```python
from build123d import *

# Parameters (mm, degrees)
SKETCH_1_R      = 1.5
SKETCH_1_R_2    = 1
SKETCH_1_R_3    = 15
SKETCH_1_R_4    = 2.5
SKETCH_1_R_5    = 6.45
EXTRUDE_1_DEPTH = 2
FILLET_1_R      = 0.75


with BuildPart() as part:
    # 草图1 → 凸台-拉伸1 (new body)
    # profile 1 of 11: a face of its own
    with BuildSketch(Plane(origin=(0, 0, 0), x_dir=(1, 0, 0), z_dir=(0, 1, 0))):
        Polygon((-19.848034865, 26.695013128), (-30, 23), (30, 23), (19.848034865, 26.695013128), (0.026493373, 26.695013128), (-0.026493373, 26.695013128), align=None)
    # profile 2 of 11: a face of its own
    with BuildSketch(Plane(origin=(0, 0, 0), x_dir=(1, 0, 0), z_dir=(0, 1, 0))):
        Polygon((-19.848034865, 26.695013128), (-30, 23), (30, 23), (19.848034865, 26.695013128), (0.026493373, 26.695013128), (-0.026493373, 26.695013128), align=None)
    # profile 3 of 11: a face of its own
    with BuildSketch(Plane(origin=(0, 0, 0), x_dir=(1, 0, 0), z_dir=(0, 1, 0))):
        Polygon((-30, 23), (-50, 23), (-50, 7), (-50, -1), (-50, -5), (-50, -23), (-42, -23), (42, -23), (50, -23), (50, -5), (50, -1), (50, 7), (50, 23), (30, 23), align=None)
        with Locations(Location((-46, -15, 0), (0, 0, 270))):
            Circle(SKETCH_1_R, mode=Mode.SUBTRACT)
        with Locations(Location((-30.7465, -13.935, 0), (0, 0, 270))):
            Circle(SKETCH_1_R, mode=Mode.SUBTRACT)
        with Locations(Location((-12.727922061, -5.727922061, 0), (0, 0, 270))):
            Circle(SKETCH_1_R_2, mode=Mode.SUBTRACT)
        with BuildLine():
            ThreePointArc((-20.969611628, -19), (-22.969611628, -17), (-20.969611628, -15))
            Line((-20.969611628, -15), (20.969611628, -15))
            ThreePointArc((20.969611628, -15), (22.969611628, -17), (20.969611628, -19))
            Line((20.969611628, -19), (-20.969611628, -19))
        make_face(mode=Mode.SUBTRACT)
        with Locations(Location((30.7465, -13.935, 0), (0, 0, 270))):
            Circle(SKETCH_1_R, mode=Mode.SUBTRACT)
        with BuildLine():
            ThreePointArc((-6, -13), (-7.5, -11.5), (-6, -10))
            Line((-6, -10), (6, -10))
            ThreePointArc((6, -10), (7.5, -11.5), (6, -13))
            Line((6, -13), (-6, -13))
        make_face(mode=Mode.SUBTRACT)
        with Locations(Location((12.727922061, -5.727922061, 0), (0, 0, 270))):
            Circle(SKETCH_1_R_2, mode=Mode.SUBTRACT)
        with Locations(Location((46, -15, 0), (0, 0, 270))):
            Circle(SKETCH_1_R, mode=Mode.SUBTRACT)
        with Locations(Location((-46, 0, 0), (0, 0, 270))):
            Circle(SKETCH_1_R, mode=Mode.SUBTRACT)
        with Locations(Location((-46, 15, 0), (0, 0, 270))):
            Circle(SKETCH_1_R, mode=Mode.SUBTRACT)
        with Locations(Location((-30.7465, 13.935, 0), (0, 0, 270))):
            Circle(SKETCH_1_R, mode=Mode.SUBTRACT)
        with Locations(Location((-12.727922061, 19.727922061, 0), (0, 0, 270))):
            Circle(SKETCH_1_R_2, mode=Mode.SUBTRACT)
        with Locations((0, 7)):
            Circle(SKETCH_1_R_3, mode=Mode.SUBTRACT)
        with Locations(Location((46, 0, 0), (0, 0, 270))):
            Circle(SKETCH_1_R, mode=Mode.SUBTRACT)
        with Locations(Location((30.7465, 13.935, 0), (0, 0, 270))):
            Circle(SKETCH_1_R, mode=Mode.SUBTRACT)
        with Locations(Location((12.727922061, 19.727922061, 0), (0, 0, 270))):
            Circle(SKETCH_1_R_2, mode=Mode.SUBTRACT)
        with Locations(Location((46, 15, 0), (0, 0, 270))):
            Circle(SKETCH_1_R, mode=Mode.SUBTRACT)
    # profile 4 of 11: a face of its own
    with BuildSketch(Plane(origin=(0, 0, 0), x_dir=(1, 0, 0), z_dir=(0, 1, 0))):
        Polygon((-30, 23), (-50, 23), (-50, 7), (-50, -1), (-50, -5), (-50, -23), (-42, -23), (42, -23), (50, -23), (50, -5), (50, -1), (50, 7), (50, 23), (30, 23), align=None)
        with Locations(Location((-46, -15, 0), (0, 0, 270))):
            Circle(SKETCH_1_R, mode=Mode.SUBTRACT)
        with Locations(Location((-30.7465, -13.935, 0), (0, 0, 270))):
            Circle(SKETCH_1_R, mode=Mode.SUBTRACT)
        with Locations(Location((-12.727922061, -5.727922061, 0), (0, 0, 270))):
            Circle(SKETCH_1_R_2, mode=Mode.SUBTRACT)
        with BuildLine():
            ThreePointArc((-20.969611628, -19), (-22.969611628, -17), (-20.969611628, -15))
            Line((-20.969611628, -15), (20.969611628, -15))
            ThreePointArc((20.969611628, -15), (22.969611628, -17), (20.969611628, -19))
            Line((20.969611628, -19), (-20.969611628, -19))
        make_face(mode=Mode.SUBTRACT)
        with Locations(Location((30.7465, -13.935, 0), (0, 0, 270))):
            Circle(SKETCH_1_R, mode=Mode.SUBTRACT)
        with BuildLine():
            ThreePointArc((-6, -13), (-7.5, -11.5), (-6, -10))
            Line((-6, -10), (6, -10))
            ThreePointArc((6, -10), (7.5, -11.5), (6, -13))
            Line((6, -13), (-6, -13))
        make_face(mode=Mode.SUBTRACT)
        with Locations(Location((12.727922061, -5.727922061, 0), (0, 0, 270))):
            Circle(SKETCH_1_R_2, mode=Mode.SUBTRACT)
        with Locations(Location((46, -15, 0), (0, 0, 270))):
            Circle(SKETCH_1_R, mode=Mode.SUBTRACT)
        with Locations(Location((-46, 0, 0), (0, 0, 270))):
            Circle(SKETCH_1_R, mode=Mode.SUBTRACT)
        with Locations(Location((-46, 15, 0), (0, 0, 270))):
            Circle(SKETCH_1_R, mode=Mode.SUBTRACT)
        with Locations(Location((-30.7465, 13.935, 0), (0, 0, 270))):
            Circle(SKETCH_1_R, mode=Mode.SUBTRACT)
        with Locations(Location((-12.727922061, 19.727922061, 0), (0, 0, 270))):
            Circle(SKETCH_1_R_2, mode=Mode.SUBTRACT)
        with Locations((0, 7)):
            Circle(SKETCH_1_R_3, mode=Mode.SUBTRACT)
        with Locations(Location((46, 0, 0), (0, 0, 270))):
            Circle(SKETCH_1_R, mode=Mode.SUBTRACT)
        with Locations(Location((30.7465, 13.935, 0), (0, 0, 270))):
            Circle(SKETCH_1_R, mode=Mode.SUBTRACT)
        with Locations(Location((12.727922061, 19.727922061, 0), (0, 0, 270))):
            Circle(SKETCH_1_R_2, mode=Mode.SUBTRACT)
        with Locations(Location((46, 15, 0), (0, 0, 270))):
            Circle(SKETCH_1_R, mode=Mode.SUBTRACT)
    # profile 5 of 11: a face of its own
    with BuildSketch(Plane(origin=(0, 0, 0), x_dir=(1, 0, 0), z_dir=(0, 1, 0))):
        with Locations((0, 7)):
            Circle(SKETCH_1_R_3)
        with BuildLine():
            ThreePointArc((13, 7), (12.434860091, 3.208660592), (10.788576229, -0.253042323))
            ThreePointArc((10.788576229, -0.253042323), (9.192388155, -2.192388155), (7.253042323, -3.788576229))
            ThreePointArc((7.253042323, -3.788576229), (0, -6), (-7.253042323, -3.788576229))
            ThreePointArc((-7.253042323, -3.788576229), (-9.192388155, -2.192388155), (-10.788576229, -0.253042323))
            ThreePointArc((-10.788576229, -0.253042323), (-13, 7), (-10.788576229, 14.253042323))
            ThreePointArc((-10.788576229, 14.253042323), (-9.192388155, 16.192388155), (-7.253042323, 17.788576229))
            ThreePointArc((-7.253042323, 17.788576229), (0, 20), (7.253042323, 17.788576229))
            ThreePointArc((7.253042323, 17.788576229), (9.192388155, 16.192388155), (10.788576229, 14.253042323))
            ThreePointArc((10.788576229, 14.253042323), (12.434860091, 10.791339408), (13, 7))
        make_face(mode=Mode.SUBTRACT)
    # profile 6 of 11: a face of its own
    with BuildSketch(Plane(origin=(0, 0, 0), x_dir=(1, 0, 0), z_dir=(0, 1, 0))):
        with BuildLine():
            ThreePointArc((7.253042323, -3.788576229), (9.192388155, -2.192388155), (10.788576229, -0.253042323))
            Line((10.788576229, -0.253042323), (4.242640687, 6.292893219))
            ThreePointArc((4.242640687, 6.292893219), (3.949747468, 7), (4.242640687, 7.707106781))
            Line((4.242640687, 7.707106781), (10.788576229, 14.253042323))
            ThreePointArc((10.788576229, 14.253042323), (9.192388155, 16.192388155), (7.253042323, 17.788576229))
            Line((7.253042323, 17.788576229), (0.707106781, 11.242640687))
            ThreePointArc((0.707106781, 11.242640687), (0, 10.949747468), (-0.707106781, 11.242640687))
            Line((-0.707106781, 11.242640687), (-7.253042323, 17.788576229))
            ThreePointArc((-7.253042323, 17.788576229), (-9.192388155, 16.192388155), (-10.788576229, 14.253042323))
            Line((-10.788576229, 14.253042323), (-4.242640687, 7.707106781))
            ThreePointArc((-4.242640687, 7.707106781), (-3.949747468, 7), (-4.242640687, 6.292893219))
            Line((-4.242640687, 6.292893219), (-10.788576229, -0.253042323))
            ThreePointArc((-10.788576229, -0.253042323), (-9.192388155, -2.192388155), (-7.253042323, -3.788576229))
            Line((-7.253042323, -3.788576229), (-0.707106781, 2.757359313))
            ThreePointArc((-0.707106781, 2.757359313), (0, 3.050252532), (0.707106781, 2.757359313))
            Line((0.707106781, 2.757359313), (7.253042323, -3.788576229))
        make_face()
        with Locations(Location((-3.181980515, 3.818019485, 0), (0, 0, 270))):
            Circle(SKETCH_1_R_2, mode=Mode.SUBTRACT)
        with Locations(Location((-3.181980515, 10.181980515, 0), (0, 0, 270))):
            Circle(SKETCH_1_R_2, mode=Mode.SUBTRACT)
        with Locations(Location((3.181980515, 3.818019485, 0), (0, 0, 270))):
            Circle(SKETCH_1_R_2, mode=Mode.SUBTRACT)
        with Locations(Location((0, 7, 0), (0, 0, 270))):
            Circle(SKETCH_1_R_4, mode=Mode.SUBTRACT)
        with Locations(Location((3.181980515, 10.181980515, 0), (0, 0, 270))):
            Circle(SKETCH_1_R_2, mode=Mode.SUBTRACT)
    # profile 7 of 11: a face of its own
    with BuildSketch(Plane(origin=(0, 0, 0), x_dir=(1, 0, 0), z_dir=(0, 1, 0))):
        Polygon((42, -23), (-42, -23), (-30, -35), (30, -35), align=None)
        with BuildLine():
            ThreePointArc((-20.969611628, -31), (-22.969611628, -29), (-20.969611628, -27))
            Line((-20.969611628, -27), (20.969611628, -27))
            ThreePointArc((20.969611628, -27), (22.969611628, -29), (20.969611628, -31))
            Line((20.969611628, -31), (-20.969611628, -31))
        make_face(mode=Mode.SUBTRACT)
    # profile 8 of 11: a face of its own
    with BuildSketch(Plane(origin=(0, 0, 0), x_dir=(1, 0, 0), z_dir=(0, 1, 0))):
        Polygon((-50, -5), (-50, -1), (-58, 7), (-62, 7), align=None)
    # profile 9 of 11: a face of its own
    with BuildSketch(Plane(origin=(0, 0, 0), x_dir=(1, 0, 0), z_dir=(0, 1, 0))):
        Polygon((-50, 7), (-50, 23), (-66, 23), (-66, 7), (-62, 7), (-58, 7), align=None)
        with Locations(Location((-58, 15, 0), (0, 0, 270))):
            Circle(SKETCH_1_R_5, mode=Mode.SUBTRACT)
    # profile 10 of 11: a face of its own
    with BuildSketch(Plane(origin=(0, 0, 0), x_dir=(1, 0, 0), z_dir=(0, 1, 0))):
        Polygon((66, 23), (50, 23), (50, 7), (58, 7), (62, 7), (66, 7), align=None)
        with Locations(Location((58, 15, 0), (0, 0, 270))):
            Circle(SKETCH_1_R_5, mode=Mode.SUBTRACT)
    # profile 11 of 11: a face of its own
    with BuildSketch(Plane(origin=(0, 0, 0), x_dir=(1, 0, 0), z_dir=(0, 1, 0))):
        Polygon((58, 7), (50, -1), (50, -5), (62, 7), align=None)
    extrude(amount=EXTRUDE_1_DEPTH)

    # 圆角1
    fillet_1_edges = [part.edges().sort_by_distance(p)[0] for p in [
        (66, 1, -23),
        (66, 1, -7),
        (62, 1, -7),
        (50, 1, 5),
        (50, 1, 23),
        (42, 1, 23),
        (30, 1, 35),
        (-30, 1, 35),
        (-42, 1, 23),
        (-50, 1, 23),
        (-50, 1, 5),
        (-62, 1, -7),
        (-66, 1, -7),
        (50, 1, -7),
        (50, 1, 1),
        (58, 1, -7),
        (-50, 1, 1),
        (-50, 1, -7),
        (-58, 1, -7),
    ]]
    fillet(fillet_1_edges, radius=FILLET_1_R)


solid = part.part
```
The model under review builds one solid part; all positions refer to its coordinate system, in mm. A direction names the side the tool comes from. Round coordinates to 2 decimals unless told otherwise and drop trailing zeros. Loops run counter-clockwise (first coordinate to the right, second up) from the corner with the lowest first, then second, coordinate; pieces in that order, holes last. Notation, with made-up numbers: (50, -30) - (66, -30) arc R19 ccw to (66, 6) - close; hole circle Ø4 at (44, 19.25). An arc over 180 degrees is marked (long way). Use a Markdown table: item, result. Add a question column.
Q1. Add section A-A (x = -46). State the section outline as (y, z) points, plus the area to 3 significant figures.
Q2. Add section B-B (y = 1.5). State how many separate pieces and enclosed holes the cut face has, plus the area to 3 significant figures.
Q3. For probe 1 along Z at (x, y) = (11.5, 1.1); probe 2 along Z at (x, y) = (-30, 0.9); probe 3 along X at (y, z) = (0.5, 16), list the stretches that pass through material, from the lowest coordinate up.
Q4. Machinability: for faces 3 (the face through (-4.026, 0.986, 0.561)), 4 (the face through (56, 1, -1)), which of the approach directions +Z, -Z, +X, -X, +Y, -Y give a long, thin tool a straight path to every point of the face, cutting with its end or side? Answer none if there is none.
Q5. The part is to be moulded in two halves that separate along Z. For faces 1 (the face through (-36, 1, 29)), 2 (the face through (44.536, 0.986, -0.325)), say which applies: pulls with the +Z half, pulls with the -Z half, needs draft (parallel to the pull), parting line crosses it, or undercut.
Q6. Insertion check: pin 1 Ø1 at (x, y) = (-49, 1.5) entering from -Z; pin 2 Ø2 at (x, z) = (27.5, 17.5) entering from -Y; pin 3 Ø0.6 at (y, z) = (1, 14.5) entering from -X. Each pin has a flat end and moves straight along its axis. Give the tip position at first contact, or say it passes through.
Worked answers:
| question | item | result |
|---|---|---|
| 1 | outline | (0, -23) - (2, -23) - (2, -16.5) - (0, -16.5) - close; (0, -13.5) - (2, -13.5) - (2, -1.5) - (0, -1.5) - close; (0, 1.5) - (2, 1.5) - (2, 13.5) - (0, 13.5) - close; (0, 16.5) - (2, 16.5) - (2, 23) - (0, 23) - close |
| 1 | area | 74.0 mm² |
| 2 | separate pieces | 1 |
| 2 | enclosed holes | 30 |
| 2 | area | 5,170 mm² |
| 3 | probe 1 | -26.7 to -13.06, -0.94 to 15, 19 to 27, 31 to 35 |
| 3 | probe 2 | -23 to -15.24, -12.63 to 12.63, 15.24 to 34.93 |
| 3 | probe 3 | -50 to -47.12, -44.88 to -22.7, 22.7 to 44.88, 47.12 to 50 |
| 4 | face 3 | +Y, -Y |
| 4 | face 4 | +Z, +X, +Y, -Y |
| 5 | face 1 | pulls with the +Z half |
| 5 | face 2 | undercut |
| 6 | pin 1 | z = -23 |
| 6 | pin 2 | y = 0 |
| 6 | pin 3 | x = -50 |
